For this review, take the finished solid that the model builds, in its own axes (mm). A direction names the side the tool comes from. Give positions to 0.01 mm unless a question says otherwise; leave off trailing zeros. Write each loop counter-clockwise with the first axis right and the second up, starting at its lowest first coordinate (ties: lowest second). Pieces come first, ordered by that corner, then holes. Notation, with made-up numbers: M -17,7.5 L -11,7.5 A19 ccw -11,38.5 Z; hole C -12.75,35 d7. An arc over 180 degrees is marked long. One line per item, written item: value. Start each with the question number.
Item 1: Consider section C-C, the plane y = 3. Write out the cut boundary in (x, z), and give its area (3 significant figures).
Item 2: Consider section D-D, the plane x = 12. Write out the cut boundary in (y, z).
Item 3: Mouldability with a two-part tool opening along Z and no side actions: class faces 3 (the face through (2.54, -10.74, 2.38)), 4 (the face through (2.544, 6.446, -0.221)), 5 (the face through (19.844, -2, -4)) as released by +Z, released by -Z, zero draft, split by the parting line, or undercut.
Item 4: To check wall thickness, follow probe 1 along Y at (x, z) = (3.3, 0); probe 2 along Y at (x, z) = (11.5, 0); probe 3 along Z at (x, y) = (6, 3.25). State the ranges of each line that lie inside material, in increasing order.
Item 5: Clearance check with flat-ended pins moving along their axes: pin 1 Ø2.5 at (y, z) = (8.13, 0) entering from -X; pin 2 Ø6 at (x, z) = (9, -5) entering from -Y; pin 3 Ø6 at (x, y) = (16, 0.5) entering from +Z; pin 4 Ø3 at (x, z) = (10, 2) entering from -Y. State where each tip first meets the part, or that it passes through.
Item 6: Consider section A-A, the plane y = 0. Write out the cut boundary in (x, z), and give its area (3 significant figures).
Item 7: Tool access review of faces 1 (the face through (2.544, -6.446, 0.221)), 2 (the face through (12.4, 1.6, 5)): name each direction out of +Z, -Z, +X, -X, +Y, -Y from which nothing blocks a thin tool from reaching the whole face with its end or side.
```python
from build123d import *

# Parameters (mm, degrees)
SKETCH4_R           = 11
BOSS_EXTRUDE2_DEPTH = 5.159375
SKETCH5_R           = 5.25
BOSS_EXTRUDE3_DEPTH = 19.84375
SKETCH6_R           = 1.7
CUT_EXTRUDE1_DEPTH  = 5.159375
CIRPATTERN2_COUNT   = 4
SKETCH8_R           = 4.0005
CUT_EXTRUDE3_DEPTH  = 26.214567497


with BuildPart() as part:
    # Sketch4 → Boss-Extrude2 (new body)
    with BuildSketch(Plane(origin=(0, 0, 0), x_dir=(0, 0, -1), z_dir=(1, 0, 0))):
        Circle(SKETCH4_R)
    extrude(amount=BOSS_EXTRUDE2_DEPTH)

    # Sketch5 → Boss-Extrude3 (add)
    with BuildSketch(Plane.ZY):
        Circle(SKETCH5_R)
    extrude(amount=-BOSS_EXTRUDE3_DEPTH)

    # Sketch6 → Cut-Extrude1 (cut)
    with BuildSketch(Plane(origin=(0, 0, 0), x_dir=(0, 0, -1), z_dir=(1, 0, 0))):
        with Locations(Location((0, 8.1315, 0), (0, 0, 180))):
            Circle(SKETCH6_R)
    cut_extrude1 = extrude(amount=CUT_EXTRUDE1_DEPTH, mode=Mode.SUBTRACT)

    # CirPattern2: Cut-Extrude1 ×4 about axis
    cirpattern2_axis = Axis((0, 0, 0), (1, 0, 0))
    for i in range(1, CIRPATTERN2_COUNT):
        add(cut_extrude1.rotate(cirpattern2_axis, i * 360 / CIRPATTERN2_COUNT), mode=Mode.SUBTRACT)

    # Sketch8 → Cut-Extrude3 (cut, through all)
    with BuildSketch(Plane(origin=(19.84375, 0, 0), x_dir=(0, 0, -1), z_dir=(1, 0, 0))):
        Circle(SKETCH8_R)
    extrude(amount=-CUT_EXTRUDE3_DEPTH, mode=Mode.SUBTRACT)


solid = part.part
```
Model answer:
1. outline: M 0,-10.58 L 5.16,-10.58 L 5.16,-4.31 L 19.84,-4.31 L 19.84,-2.65 L 0,-2.65 Z; M 0,2.65 L 19.84,2.65 L 19.84,4.31 L 5.16,4.31 L 5.16,10.58 L 0,10.58 Z
1. area: 131 mm2
2. outline: C 0,0 d10.5; hole C 0,0 d8
3. face 3: split by the parting line
3. face 4: undercut
3. face 5: zero draft
4. probe 1: y = -11 to -9.83, -6.43 to -4, 4 to 6.43, 9.83 to 11
4. probe 2: y = -5.25 to -4, 4 to 5.25
4. probe 3: z = -4.12 to -2.33, 2.33 to 4.12
5. pin 1: passes through
5. pin 2: stops at y = -4.85
5. pin 3: stops at z = 5.25
5. pin 4: stops at y = -5.23
6. outline: M 0,-11 L 5.16,-11 L 5.16,-9.83 L 0,-9.83 Z; M 0,-6.43 L 5.16,-6.43 L 5.16,-5.25 L 19.84,-5.25 L 19.84,-4 L 0,-4 Z; M 0,4 L 19.84,4 L 19.84,5.25 L 5.16,5.25 L 5.16,6.43 L 0,6.43 Z; M 0,9.83 L 5.16,9.83 L 5.16,11 L 0,11 Z
6. area: 73.8 mm2
7. face 1: +X, -X
7. face 2: +X
